from build123d import *

# Parameters (mm, degrees)
F0_W          = 8.812238
F0_H          = 25.4
F1_DEPTH      = 88.9
F1_DEPTH_BACK = 88.9
F2_R          = 5.08
F3_R          = 5.08
F4_R          = 5.08
F5_R          = 5.08


with BuildPart() as f1:
    # F0 (on Top) → F1 (new body, two sides)
    with BuildSketch(Plane.XY) as f1_sk:
        with Locations((-38.162628, 17.049316)):
            Rectangle(F0_W, F0_H)
    extrude(amount=F1_DEPTH)
    extrude(f1_sk.sketch, amount=-F1_DEPTH_BACK)

    # F2
    f2_edges = [f1.edges().sort_by_distance(p)[0] for p in [
        (-42.568747, 4.349316, 0),
    ]]
    fillet(f2_edges, radius=F2_R)

    # F3
    f3_edges = [f1.edges().sort_by_distance(p)[0] for p in [
        (-42.568747, 29.749316, 0),
    ]]
    fillet(f3_edges, radius=F3_R)

    # F4
    f4_edges = [f1.edges().sort_by_distance(p)[0] for p in [
        (-42.568747, 17.049316, 88.9),
    ]]
    fillet(f4_edges, radius=F4_R)

    # F5
    f5_edges = [f1.edges().sort_by_distance(p)[0] for p in [
        (-42.568747, 17.049316, -88.9),
    ]]
    fillet(f5_edges, radius=F5_R)


solid = f1.part
Verification items for the finished model (mm, model axes). Give positions to 0.01 mm unless a question says otherwise; leave off trailing zeros. Loops run counter-clockwise (first coordinate to the right, second up) from the corner with the lowest first, then second, coordinate; pieces in that order, holes last. Notation, with made-up numbers: (-19.5, 34) - (36.5, 34) arc R9 cw to (36.5, 43) - close; hole circle Ø1 at (33.25, 43). An arc over 180 degrees is marked (long way). Write item = value, one per line. Start each with the question number.
Q1. Cross-section at A-A, the plane z = 26. Enter the section's corners in (x, y).
Q2. Thickness scan on line 1 (Y direction, x = -38, z = 63.5); line 2 (Y direction, x = -40.75, z = 33); line 3 (Z direction, x = -39.5, y = 26.5). Record the ranges inside material, lowest first.
Q3. Depth check by flat-ended pin: P1, Ø4, axis at x = -39.5, z = -41.5, coming from the -Y side; P2, Ø2, axis at x = -35, y = 26, coming from the -Z side; P3, Ø2, axis at x = -39, z = 16.5, coming from the +Y side; P4, Ø1, axis at y = 8, z = 53.5, coming from the -X side. Enter the tip coordinate at first touch or a pass-through.
Q4. Cross-section at B-B, the plane x = -41. Enter the section's corners in (y, z), and give its area (3 significant figures).
Answer key:
q1.outline = (-42.57, 9.43) arc R5.08 ccw to (-37.49, 4.35) - (-33.76, 4.35) - (-33.76, 29.75) - (-37.49, 29.75) arc R5.08 ccw to (-42.57, 24.67) - close
q2.line_1 = 4.38 to 29.72
q2.line_2 = 5.53 to 28.56
q2.line_3 = -88.11 to 88.11
q3.P1 = 4.35
q3.P2 = -88.89
q3.P3 = 29.72
q3.P4 = -42.48
q4.outline = (5.76, -83.82) arc R3.67 ccw to (9.43, -87.49) - (24.67, -87.49) arc R3.67 ccw to (28.34, -83.82) - (28.34, 83.82) arc R3.67 ccw to (24.67, 87.49) - (9.43, 87.49) arc R3.67 ccw to (5.76, 83.82) - close
q4.area = 3,940 mm^2
